Autodesk Fusion 360 part; units mm, degrees
sketch "Boceto5" plane through (-11.25, 0, 0) normal (-1, 0, 0) x (0, -1, 0)
sketch "Boceto8" plane through (12.75, 0, 0) normal (1, 0, 0) x (0, 1, 0)
  line L0 (-15.65, 0) -> (-25.65, 0)
  line L1 (-25.65, 0) -> (-25.65, -18.8)
  line L2 (-25.65, -18.8) -> (-15.65, -18.8)
  line L3 (-15.65, -18.8) -> (-15.65, 0)
  line L4 (-25.65, 0) -> (-25.65, 1.5)
  line L5 (-25.65, 1.5) -> (-15.65, 1.5)
  line L6 (-15.65, 1.5) -> (-15.65, 0)
  dimension "d15" = 1.5
sketch "Boceto10" plane through (0, -25.65, 0) normal (0, -1, 0) x (1, 0, 0)
  line L0 (12.75, 0) -> (12.75, 1.5)
  line L1 (12.75, 1.5) -> (-12.75, 1.5)
  line L2 (-12.75, 1.5) -> (-12.75, 0)
  line L3 (-12.75, 0) -> (12.75, 0)
  line L4 (-12.75, 0) -> (-12.75, 1.5)
  line L5 (12.75, 1.5) -> (-12.75, 1.5)
  line L6 (12.75, 1.5) -> (12.75, 0)
  line L7 (11.25, -18.8) -> (12.75, 0)
  line L8 (11.25, -18.8) -> (12.75, 0)
  line L9 (-12.75, 0) -> (12.75, 0)
  line L10 (-11.25, -18.8) -> (-12.75, 0)
  line L11 (-11.25, -18.8) -> (-12.75, 0)
sketch "Boceto11" plane through (11.25, 0, 0) normal (1, 0, 0) x (0, 1, 0)
  line L0 (-25.65, -10.05) -> (-25.65, -18.8)
  line L1 (-25.65, -18.8) -> (7.2, -18.8)
  line L2 (7.2, -18.8) -> (7.2, 0)
  line L3 (7.2, 0) -> (-25.65, 0)
  line L4 (-25.65, 0) -> (-25.65, -10.05)
  line L5 (-24.65, 0) -> (-16.65, 0)
  line L6 (-24.65, 0) -> (-24.65, -18.8)
  line L7 (-16.65, 0) -> (-16.65, -18.8)
  dimension "d22" = 1
  dimension "d23" = 8
extrude "Extruir7" add sketch "Boceto11" along normal blind 1.5 contours L1 L3 L5 L6 L7
sketch "Boceto12" plane through (12.75, 0, 0) normal (1, 0, 0) x (0, 1, 0)
  line L0 (-24.65, 0) -> (-24.65, -18.8)
  line L1 (-24.65, -18.8) -> (-16.65, -18.8)
  line L2 (-16.65, -18.8) -> (-16.65, 0)
  line L3 (-16.65, 0) -> (-24.65, 0)
  line L4 (-24.65, 0) -> (-24.65, 1.5)
  line L5 (-16.65, 0) -> (-16.65, 1.5)
  line L6 (-16.65, 1.5) -> (-24.65, 1.5)
  dimension "d26" = 1.5
  dimension "d27" = 1.5
extrude "Extruir8" add sketch "Boceto12" against normal blind 25.5 contours L3 L4 L5 L6
sketch "Boceto13" plane through (0, 0, 0) normal (0, 0, -1) x (1, 0, 0)
  line L0 (11.25, 16.65) -> (11.25, 24.65)
  line L1 (11.25, 24.65) -> (-12.75, 24.65)
  line L2 (-12.75, 24.65) -> (-12.75, 16.65)
  line L3 (-12.75, 16.65) -> (11.25, 16.65)
  line L4 (-12.75, 24.65) -> (-11.25, 24.65)
  line L5 (-12.75, 24.65) -> (-12.75, 16.65)
  line L6 (-12.75, 16.65) -> (-11.25, 16.65)
  line L7 (-11.25, 16.65) -> (-11.25, 24.65)
  dimension "d30" = 1.5
  dimension "d31" = 1.5
extrude "Extruir9" add sketch "Boceto13" along normal blind 18.8 contours L1 L2 L3 L4 L5 L6 L7
sketch "Boceto14" plane through (0, 0, -18.8) normal (0, 0, -1) x (1, 0, 0)
  line L0 (-7.25, -11.2) -> (7.25, -11.2)
  arc A0 (7.25, -11.2) -> (11.25, -7.2) centre (7.25, -7.2) ccw
  line L1 (11.25, -7.2) -> (11.25, 25.65)
  line L2 (11.25, 25.65) -> (7.0711, 25.65)
  line L3 (7.0711, 25.65) -> (7.0711, 37.15)
  line L4 (7.0711, 37.15) -> (-7.0711, 37.15)
  line L5 (-7.0711, 37.15) -> (-7.0711, 25.65)
  line L6 (-7.0711, 25.65) -> (-11.25, 25.65)
  line L7 (-11.25, 25.65) -> (-11.25, -7.2)
  arc A1 (-11.25, -7.2) -> (-7.25, -11.2) centre (-7.25, -7.2) ccw
  circle A2 centre (8.75, 20.6) radius 1.5
  circle A3 centre (-8.75, 20.6) radius 1.5
  circle A4 centre (0, 0) radius 2.7
  line L8 (-2.5, 31.15) -> (-2.5, 32.8199)
  line L9 (-2.5, 32.8199) -> (2.5, 32.8199)
  line L10 (2.5, 32.8199) -> (2.5, 31.15)
  line L11 (2.5, 31.15) -> (-2.5, 31.15)
  circle A5 centre (8.75, 20.6) radius 1.5
extrude "Extruir10" cut sketch "Boceto14" against normal blind 25 contours A2 A5 | A3
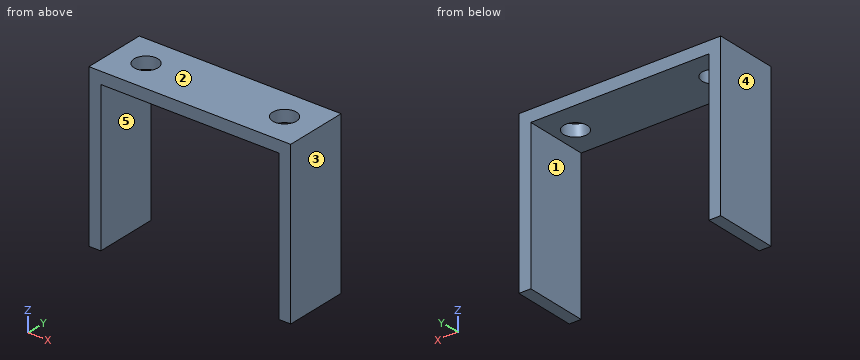
Work out the finished part from the listing and answer in its coordinate system (mm). Face numbers are marked on the shaded views. A direction names the side the tool comes from. Round coordinates to 2 decimals unless told otherwise and drop trailing zeros. Order: outer loops, then holes, each group sorted by start corner. A loop starts at its lowest first (then second) coordinate and runs counter-clockwise, first axis right, second up. Notation, with made-up numbers: M 11.5,66.25 L 61.5,66.25 A27 ccw 61.5,103.25 Z; hole C 50,66.25 d5. An arc over 180 degrees is marked long. Put each result on its own line as item: value. Start each with the question number.
Q1. Section B-B, the plane z = -13.75 is taken. Write down the section's boundary in (x, y), and give its area (3 significant figures).
Q2. For a pull along X with two mould halves and no side action, classify the marked faces 1, 2 and 3 as pulls with the +X half, pulls with the -X half, needs draft (parallel to the pull), parting line crosses it, or undercut.
Q3. Flat-ended cylindrical pins translate along their axes: pin 1 (5 mm diameter, centred on x = -6.5, z = -10.5, fed in from +Y); pin 2 (2.5 mm diameter, centred on x = 4, y = -19.5, fed in from -Z). Find the tip coordinate at first contact, or state that the pin passes through.
Q4. Section A-A, the plane y = -20.6 is taken. Write down the section's boundary in (x, z).
Q5. A tool of negligible diameter and unlimited length cuts with its end or side. For the marked faces 4 and 5, from which of +Z, -Z, +X, -X, +Y, -Y can it reach the whole face along a straight path? Write none if from no direction.
Q6. Section C-C, the plane x = -8.75 is taken. Write down the section's boundary in (y, z).
Q7. Section D-D, the plane y = -17.5 is taken. Write down the section's boundary in (x, z).
Q8. Straight lines are drawn through the part: L1, parallel to X at y = -20.6, z = 0.7; L2, parallel to Y at x = 8.75, z = 1.05; L3, parallel to X at y = -21, z = -12.75. For each, find the intervals that lie inside material, in ascending order. Write a range as [from, to].
Findings below:
1. outline: M -12.75,-24.65 L -11.25,-24.65 L -11.25,-16.65 L -12.75,-16.65 Z; M 11.25,-24.65 L 12.75,-24.65 L 12.75,-16.65 L 11.25,-16.65 Z
1. area: 24.0 mm^2
2. face 1: undercut
2. face 2: needs draft
2. face 3: pulls with the +X half
3. pin 1: passes through
3. pin 2: stops at z = 0
4. outline: M -12.75,-18.8 L -11.25,-18.8 L -11.25,0 L -10.25,0 L -10.25,1.5 L -12.75,1.5 Z; M -7.25,0 L 7.25,0 L 7.25,1.5 L -7.25,1.5 Z; M 10.25,0 L 11.25,0 L 11.25,-18.8 L 12.75,-18.8 L 12.75,1.5 L 10.25,1.5 Z
5. face 4: +Z, -Z, -X, +Y, -Y
5. face 5: -Z, +Y, -Y
6. outline: M -24.65,0 L -22.1,0 L -22.1,1.5 L -24.65,1.5 Z; M -19.1,0 L -16.65,0 L -16.65,1.5 L -19.1,1.5 Z
7. outline: M -12.75,-18.8 L -11.25,-18.8 L -11.25,0 L 11.25,0 L 11.25,-18.8 L 12.75,-18.8 L 12.75,1.5 L -12.75,1.5 Z
8. L1: x = [-12.75, -10.25], [-7.25, 7.25], [10.25, 12.75]
8. L2: y = [-24.65, -22.1], [-19.1, -16.65]
8. L3: x = [-12.75, -11.25], [11.25, 12.75]
